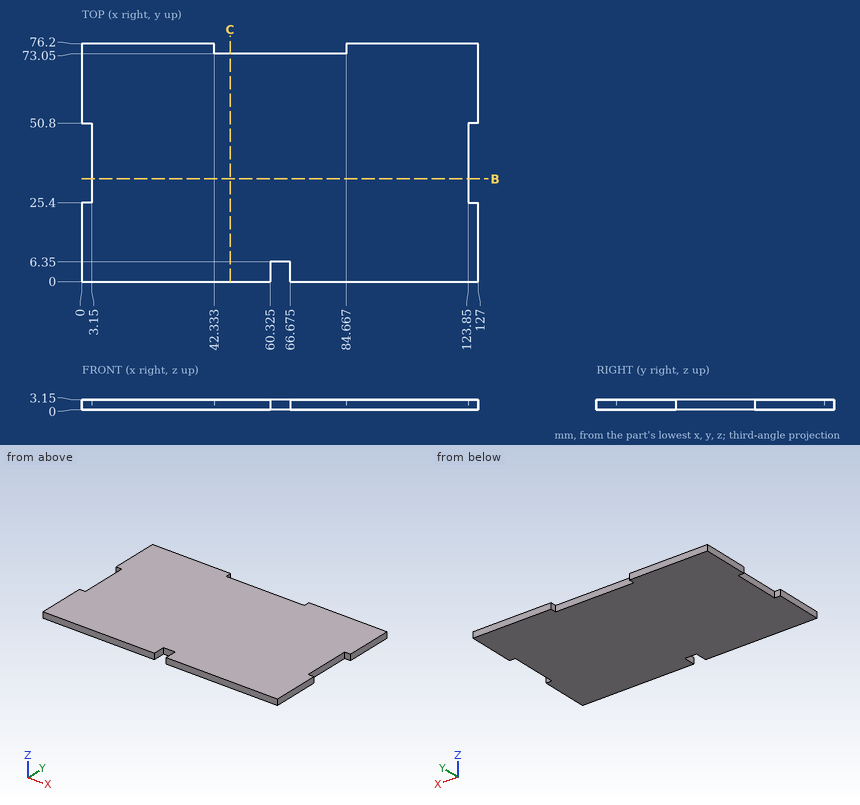
Source: three-view drawing plus pictorial views. Frame: mm from the lowest corner of the part. Round coordinates to 2 decimals unless told otherwise and drop trailing zeros. Loops run counter-clockwise (first coordinate to the right, second up) from the corner with the lowest first, then second, coordinate; pieces in that order, holes last.
Q1. Section C-C, the plane x = 47.5. Return loops of the section in (y, z).
Q2. First-contact query: P1, Ø0.9, axis at y = 2.5, z = 1.5, coming from the -X side; P2, Ø1.6, axis at x = 66, z = 2, coming from the +Y side; P3, Ø0.9, axis at x = 64.5, z = 2.5, coming from the -Y side. Flat tips, straight axial feed; report the tip coordinate or a pass-through.
Q3. Section B-B, the plane y = 33. Return loops of the section in (x, z).
Q4. Ray query, line 1 (Y direction, x = 58, z = 2.35); line 2 (Y direction, x = 63.5, z = 2.2); line 3 (X direction, y = 48, z = 3). Return the intervals inside material, ascending.
Solutions:
1. outline: (0, 0) - (73.05, 0) - (73.05, 3.15) - (0, 3.15) - close
2. P1: stops at x = 0
2. P2: stops at y = 73.05
2. P3: stops at y = 6.35
3. outline: (3.15, 0) - (123.85, 0) - (123.85, 3.15) - (3.15, 3.15) - close
4. line 1: y = 0 to 73.05
4. line 2: y = 6.35 to 73.05
4. line 3: x = 3.15 to 123.85
